The listing builds one solid part. Answer for the finished solid, in the listing's coordinates (mm). A direction names the side the tool comes from. Coordinates: 2 decimals unless noted, no trailing zeros. Order: outer loops, then holes, each group sorted by start corner. A loop starts at its lowest first (then second) coordinate and runs counter-clockwise, first axis right, second up.
```python
from build123d import *

# Parameters (mm, degrees)
EXTRUDE_N_DEPTH        = 15
EXTRUDE_START          = -15
EXTRUDE_1247_DEPTH     = 15
FILLET_1323_R          = 5
FILLET_1704_R          = 10
SKETCH_1866_R          = 1.5
CUT_EXTRUDE_1874_DEPTH = 205.73302307


# Read off the part's stored shape, not the designer's step: Крепёж подсветки
with BuildPart() as part:
    # Эскиз n → n (new body)
    with BuildSketch(Plane(origin=(0, 0, 0), x_dir=(1, 0, 0), z_dir=(0, 1, 0))):
        with BuildLine():
            Line((0, 153.846153846), (39.299935897, 153.846153846))
            Line((39.299935897, 153.846153846), (39.299935897, 146.547635651))
            ThreePointArc((39.299935897, 146.547635651), (42.668493546, 141.821284431), (48.235294238, 143.463327831))
            add(Edge.make_bspline(
                [(48.235294238, 143.463327831), (48.680235544, 144.031041426), (49.805362072, 145.350365147), (51.780881441, 147.296733708), (54.221156894, 149.205536006), (56.895496579, 150.901537566), (59.76640372, 152.374012934), (62.852222566, 153.625097643), (66.119942525, 154.659854718), (69.589237805, 155.463125454), (74.594167261, 156.227638993), (78.47972692, 156.380969617), (81.126858974, 156.41025641)],
                knots=[0.312672271, 0.312672271, 0.312672271, 0.312672271, 0.353305114, 0.410247876, 0.468663539, 0.527537938, 0.588459477, 0.650230395, 0.714969493, 0.781418224, 0.850708434, 1, 1, 1, 1], degree=3))
            add(Edge.make_bspline(
                [(81.126858974, 156.41025641), (84.859720001, 156.426218167), (90.317082636, 155.957777721), (97.302679405, 154.400552389), (102.070561998, 152.693026297), (106.574200345, 150.583974492), (110.703488298, 147.904651559), (114.548128603, 144.805781264), (118.036996775, 141.222819891), (121.14631588, 137.227946624), (123.864208469, 132.851585446), (126.126383474, 128.112461575), (128.040546504, 123.027665479), (129.455521339, 117.556714971), (130.87166816, 109.597055945), (131.274075332, 103.391251973), (131.247051282, 99.158653846)],
                knots=[0, 0, 0, 0, 0.129841575, 0.189943736, 0.248604894, 0.305783081, 0.362648635, 0.419493286, 0.477347716, 0.536300993, 0.595380588, 0.656296956, 0.718809931, 0.784206619, 0.852684575, 1, 1, 1, 1], degree=3))
            Line((131.247051282, 99.158653846), (131.247051282, 0))
            Line((131.247051282, 0), (89.700576923, 0))
            Line((89.700576923, 0), (89.700576923, 94.991987179))
            add(Edge.make_bspline(
                [(89.700576923, 94.991987179), (89.724152638, 98.525793473), (89.038605734, 103.707632052), (86.189788042, 109.795689468), (83.284125509, 113.481677505), (79.754151619, 116.49899904), (73.94336902, 119.402249568), (68.995321139, 120.166486998), (65.622051282, 120.112179487)],
                knots=[0, 0, 0, 0, 0.270259745, 0.391050185, 0.508669627, 0.625837927, 0.742508846, 1, 1, 1, 1], degree=3))
            add(Edge.make_bspline(
                [(65.622051282, 120.112179487), (62.246048707, 120.173531263), (57.293638347, 119.387703313), (51.452904124, 116.499817419), (47.884444323, 113.49367552), (44.967404733, 109.804274849), (42.196227012, 103.687541079), (41.462060906, 98.533886415), (41.503461538, 94.991987179)],
                knots=[0, 0, 0, 0, 0.257168251, 0.374600508, 0.492402658, 0.609874601, 0.73007917, 1, 1, 1, 1], degree=3))
            Line((41.503461538, 94.991987179), (41.503461538, 0))
            Line((41.503461538, 0), (0, 0))
            Line((0, 0), (0, 153.846153846))
        make_face()
    extrude(amount=EXTRUDE_N_DEPTH)

    # Extrude 1247 outline → Extrude 1247 (add)
    with BuildSketch(Plane(origin=(0, 0, 0), x_dir=(1, 0, 0), z_dir=(0, 1, 0)).offset(EXTRUDE_START)):
        with BuildLine():
            Line((15.751731, 10), (25.751731, 10))
            Line((25.751731, 10), (25.751731, 113.28080684))
            Line((25.751731, 113.28080684), (65.409736151, 130.790882853))
            ThreePointArc((65.409736151, 130.790882853), (92.515549907, 128.594316344), (105.473237, 104.685146786))
            Line((105.473237, 104.685146786), (105.473237, 10))
            Line((105.473237, 10), (115.473237, 10))
            Line((115.473237, 10), (115.473237, 104.685146786))
            ThreePointArc((115.473237, 104.685146786), (97.974906411, 136.97258744), (61.370650839, 139.938876614))
            Line((61.370650839, 139.938876614), (25.751731, 124.212165411))
            Line((25.751731, 124.212165411), (25.751731, 143.85))
            Line((25.751731, 143.85), (15.751731, 143.85))
            Line((15.751731, 143.85), (15.751731, 10))
        make_face()
    extrude(amount=EXTRUDE_1247_DEPTH)

    # Fillet 1323
    fillet_1323_edges = [part.edges().sort_by_distance(p)[0] for p in [
        (25.751731, -7.5, -143.85),
        (15.751731, -7.5, -143.85),
        (15.751731, -7.5, -10),
        (25.751731, -7.5, -10),
        (105.473237, -7.5, -10),
        (115.473237, -7.5, -10),
    ]]
    fillet(fillet_1323_edges, radius=FILLET_1323_R - 0.0001)  # a hair under: the kernel refuses the full size

    # Fillet 1704
    fillet_1704_edges = [part.edges().sort_by_distance(p)[0] for p in [
        (25.751731, -7.5, -124.212165411),
        (25.751731, -7.5, -113.28080684),
    ]]
    fillet(fillet_1704_edges, radius=FILLET_1704_R)

    # Sketch 1866 → Cut-Extrude 1874 (cut, through all)
    with BuildSketch(Plane(origin=(0, 0, 0), x_dir=(1, 0, 0), z_dir=(0, 1, 0))):
        with Locations(Location((98.28, 130.55, 0), (0, 0, 270))):
            Circle(SKETCH_1866_R)
        with Locations(Location((20.751731, 15, 0), (0, 0, 270))):
            Circle(SKETCH_1866_R)
        with Locations(Location((110.473237, 15, 0), (0, 0, 270))):
            Circle(SKETCH_1866_R)
    extrude(amount=-CUT_EXTRUDE_1874_DEPTH, mode=Mode.SUBTRACT)


solid = part.part
```
1) A cutting plane is placed at C-C, the plane y = -4.5. Count the separate pieces of the cut face and the enclosed holes in it, plus the area to 3 significant figures.
2) A cutting plane is placed at A-A, the plane z = -21.5. Write down the section's boundary in (x, y), plus the area to 3 significant figures.
3) The mould has two halves that part along X. Classify faces 4 (the cylindrical face through (106.977, -7.395, -11.426)), 5 (the flat face through (19, 7, -153.846)), 6 (the cylindrical face through (17.18, -7.4, -11.5)), 7 (the flat face through (115.473, -8, -59)): released by +X, released by -X, zero draft, split by the parting line, or undercut.
4) For faces 1 (the flat face through (41.503, 7, -48)), 2 (the flat face through (37, 0, -79)), 3 (the flat face through (105.473, -8, -60)), determine the directions among +Z, -Z, +X, -X, +Y, -Y from which every point of the face is accessible in a straight line to the end or side of a thin tool.
5) Straight lines are drawn through the part: probe 1 along X at (y, z) = (-9, -15); probe 2 along X at (y, z) = (-10, -59.5); probe 3 along Y at (x, z) = (111.5, -126.5). For each, find the intervals that lie inside material, in ascending order.
6) Each of these flat-tipped pins is pushed along its axis until it touches: P1, Ø12, axis at x = 25, y = -8.5, coming from the -Z side; P2, Ø4.5, axis at y = -5, z = -90.5, coming from the -X side; P3, Ø2.5, axis at x = 20.75, z = -15, coming from the -Y side. Where does it stop, or does it pass through?
7) A cutting plane is placed at B-B, the plane x = 10. Write down the section's boundary in (y, z), plus the area to 3 significant figures.
Working result:
1. separate pieces: 1
1. enclosed holes: 3
1. area: 3,370 mm2
2. outline: (0, 0) - (15.75, 0) - (15.75, -15) - (25.75, -15) - (25.75, 0) - (41.5, 0) - (41.5, 15) - (0, 15) - close; (89.7, 0) - (105.47, 0) - (105.47, -15) - (115.47, -15) - (115.47, 0) - (131.25, 0) - (131.25, 15) - (89.7, 15) - close
2. area: 1,550 mm2
3. face 4: undercut
3. face 5: zero draft
3. face 6: released by -X
3. face 7: released by +X
4. face 1: +Z, +Y, -Y
4. face 2: -Y
4. face 3: +Z, -Y
5. probe 1: x = 15.75 to 19.25, 22.25 to 25.75, 105.47 to 108.97, 111.97 to 115.47
5. probe 2: x = 15.75 to 25.75, 105.47 to 115.47
5. probe 3: y = 0 to 15
6. P1: stops at z = -143.85
6. P2: stops at x = 15.75
6. P3: stops at y = 0
7. outline: (0, -153.85) - (15, -153.85) - (15, 0) - (0, 0) - close
7. area: 2,310 mm2
